```python
from build123d import *

# Parameters (mm, degrees)
SKETCH2_R          = 114.3
SKETCH2_R_2        = 31.75
EXTRUDE1_DEPTH     = 6.35
CUT_EXTRUDE1_REACH = 163.769
SKETCH3_R          = 8.5328125


with BuildPart() as part:
    # Sketch2 → Extrude1 (new body)
    with BuildSketch(Plane.XY):
        Circle(SKETCH2_R)
        Circle(SKETCH2_R_2, mode=Mode.SUBTRACT)
    extrude(amount=EXTRUDE1_DEPTH)

    # Sketch3 → Cut-Extrude1 (cut, up to next)
    with BuildSketch(Plane.XY.offset(6.35), mode=Mode.PRIVATE) as cut_extrude1_sk1:
        with Locations((-65.0875, -65.0875)):
            Circle(SKETCH3_R)
    cut_extrude1_tool1 = extrude(cut_extrude1_sk1.sketch, amount=-CUT_EXTRUDE1_REACH, mode=Mode.PRIVATE) & part.part
    # Sketch3 → Cut-Extrude1 (cut, up to next)
    with BuildSketch(Plane.XY.offset(6.35), mode=Mode.PRIVATE) as cut_extrude1_sk2:
        with Locations((-65.0875, 65.0875)):
            Circle(SKETCH3_R)
    cut_extrude1_tool2 = extrude(cut_extrude1_sk2.sketch, amount=-CUT_EXTRUDE1_REACH, mode=Mode.PRIVATE) & part.part
    # Sketch3 → Cut-Extrude1 (cut, up to next)
    with BuildSketch(Plane.XY.offset(6.35), mode=Mode.PRIVATE) as cut_extrude1_sk3:
        with Locations((65.0875, 65.0875)):
            Circle(SKETCH3_R)
    cut_extrude1_tool3 = extrude(cut_extrude1_sk3.sketch, amount=-CUT_EXTRUDE1_REACH, mode=Mode.PRIVATE) & part.part
    # Sketch3 → Cut-Extrude1 (cut, up to next)
    with BuildSketch(Plane.XY.offset(6.35), mode=Mode.PRIVATE) as cut_extrude1_sk4:
        with Locations((65.0875, -65.0875)):
            Circle(SKETCH3_R)
    cut_extrude1_tool4 = extrude(cut_extrude1_sk4.sketch, amount=-CUT_EXTRUDE1_REACH, mode=Mode.PRIVATE) & part.part
    add(cut_extrude1_tool1.solids().sort_by_distance((-65.0875, -65.0875, 6.35))[0], mode=Mode.SUBTRACT)
    add(cut_extrude1_tool2.solids().sort_by_distance((-65.0875, 65.0875, 6.35))[0], mode=Mode.SUBTRACT)
    add(cut_extrude1_tool3.solids().sort_by_distance((65.0875, 65.0875, 6.35))[0], mode=Mode.SUBTRACT)
    add(cut_extrude1_tool4.solids().sort_by_distance((65.0875, -65.0875, 6.35))[0], mode=Mode.SUBTRACT)


solid = part.part
```
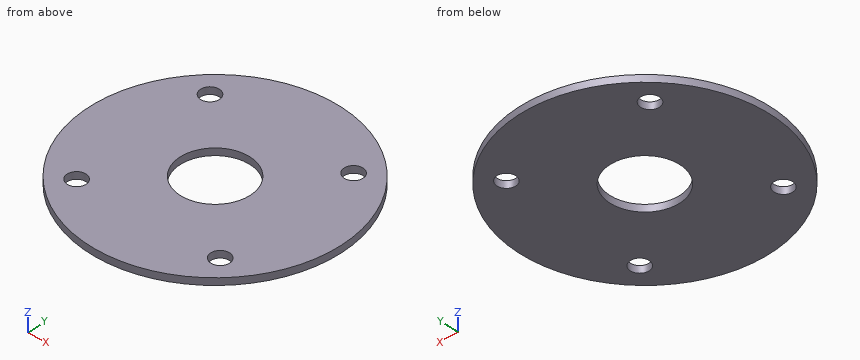
Here's how the part is built. I have some questions about the finished solid (model axes, mm). Round coordinates to 2 decimals unless told otherwise and drop trailing zeros. Order: outer loops, then holes, each group sorted by start corner. A loop starts at its lowest first (then second) coordinate and runs counter-clockwise, first axis right, second up. Notation, with made-up numbers: M 70,-31 L 118,-31 A28 cw 118,-5 Z; hole C 3,-7.5 d8. An arc over 180 degrees is marked long. Use CSV: the item, a comma, the result in double quotes.
1) I want a section at C-C (z = 3). List the corners of the cut face in (x, y) for me.
Taken from the geometry:
outline,"C 0,0 d228.6; hole C -65.09,-65.09 d17.07; hole C -65.09,65.09 d17.07; hole C 0,0 d63.5; hole C 65.09,-65.09 d17.07; hole C 65.09,65.09 d17.07"
2) I want a section at D-D (y = -40). List the corners of the cut face in (x, z) for me, then the cut area to 3 significant figures.
Taken from the geometry:
outline,"M -107.07,0 L 107.07,0 L 107.07,6.35 L -107.07,6.35 Z"
area,"1,360 mm^2"
3) I'm going to push flat-ended pins straight in: P1, Ø1.5, axis at y = -39, z = 2.5, coming from the +X side; P2, Ø3, axis at y = 63.5, z = 4.5, coming from the -X side. Where does each tip first touch, or does it pass through?
Taken from the geometry:
P1,"x = 107.71"
P2,"x = -96.02"
4) I need wall thicknesses on line 1 along Y through (x, z) = (0, 4); line 2 along Y through (x, z) = (8, 3.75); line 3 along X through (y, z) = (-71.5, 1.25). Which ranges of each line are inside material? Lowest first, please. Write a range as [from, to].
Taken from the geometry:
line 1,"[-114.3, -31.75], [31.75, 114.3]"
line 2,"[-114.02, -30.73], [30.73, 114.02]"
line 3,"[-89.18, -70.72], [-59.46, 59.46], [70.72, 89.18]"
5) I want a section at A-A (x = 0). List the corners of the cut face in (y, z) for me, then the cut area to 3 significant figures.
Taken from the geometry:
outline,"M -114.3,0 L -31.75,0 L -31.75,6.35 L -114.3,6.35 Z; M 31.75,0 L 114.3,0 L 114.3,6.35 L 31.75,6.35 Z"
area,"1,050 mm^2"
